Design review of the part built by this model. Coordinates are the model's own, in mm. Face numbers are marked on the shaded views. A direction names the side the tool comes from. Give positions to 0.01 mm unless a question says otherwise; leave off trailing zeros. Order: outer loops, then holes, each group sorted by start corner. A loop starts at its lowest first (then second) coordinate and runs counter-clockwise, first axis right, second up. Notation, with made-up numbers: (60, 34.25) -> (84, 34.25) arc R15 cw to (84, 54.25) -> close; hole circle Ø2 at (-39.75, 46.25). An arc over 180 degrees is marked (long way). Answer in a Markdown table with one row per item. Add a question column.
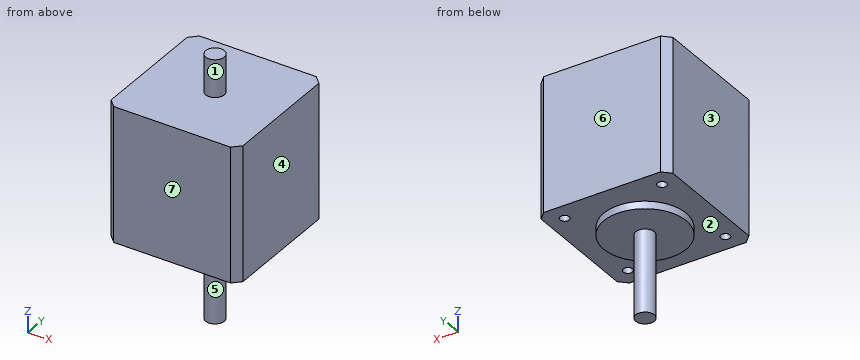
Solid Edge part; units mm, degrees
sketch "Sketch1" plane through (0, 0, 0) normal (0, 0, 1) x (1, 0, 0)
  circle A0 centre (0, 0) radius 2.5
extrude "Protrusion1" add sketch "Sketch1" along normal blind 24
sketch "Sketch2" plane through (0, 0, 24) normal (0, 0, 1) x (1, 0, 0)
  circle A0 centre (0, 0) radius 11
extrude "ExtrudedProtrusion_2" add sketch "Sketch2" against normal blind 2
sketch "Sketch3" plane through (0, 0, 24) normal (0, 0, 1) x (1, 0, 0)
  line L0 (-15.6, -17.6) -> (15.6, -17.6)
  line L1 (15.6, -17.6) -> (17.6, -15.6)
  line L2 (17.6, -15.6) -> (17.6, 15.6)
  line L3 (15.6, 17.6) -> (17.6, 15.6)
  line L4 (15.6, 17.6) -> (-15.6, 17.6)
  line L5 (-15.6, 17.6) -> (-17.6, 15.6)
  line L6 (-17.6, 15.6) -> (-17.6, -15.6)
  line L7 (-15.6, -17.6) -> (-17.6, -15.6)
extrude "ExtrudedProtrusion_3" add sketch "Sketch3" along normal blind 36
hole "Hole_1" at (-13, -13, 24) direction (0, 0, 1) diameter 2.459 depth 2.5 thread major 3 thread length 2.5
hole "Hole1" at (-13, 13, 24) direction (0, 0, 1) diameter 2.459 depth 2.5 thread major 3 thread length 2.5
hole "Hole2" at (13, 13, 24) direction (0, 0, 1) diameter 2.459 depth 2.5 thread major 3 thread length 2.5
hole "Hole3" at (13, -13, 24) direction (0, 0, 1) diameter 2.459 depth 2.5 thread major 3 thread length 2.5
sketch "Sketch4" plane through (0, 0, 60) normal (0, 0, 1) x (1, 0, 0)
  circle A0 centre (0, 0) radius 2.5
extrude "ExtrudedProtrusion_4" add sketch "Sketch4" along normal blind 10
1) Add section A-A, the plane x = -13. Write out the cut boundary in (y, z).
2) Clearance check with flat-ended pins moving along their axes: P1, Ø3, axis at x = 13, y = 13, coming from the -Z side; P2, Ø6.5, axis at x = 2, y = -3, coming from the -Z side; P3, Ø2, axis at x = -13, y = 13, coming from the +Z side; P4, Ø1.2, axis at x = 13, y = -13.5, coming from the -Z side. State where each tip first meets the part, or that it passes through.
3) Machinability: for the marked faces 1, 2 and 3, which of the approach directions +Z, -Z, +X, -X, +Y, -Y give a long, thin tool a straight path to every point of the face, cutting with its end or side? Answer none if there is none.
4) For L1, parallel to X at y = -13, z = 25.25; L2, parallel to Z at x = -13.5, y = 14.5, list the stretches that pass through material, from the lowest coordinate up.
5) Mouldability with a two-part tool opening along Y and no side actions: class the marked faces 4, 5, 6 and 7 as +Y half, -Y half, draft (parallel to the pull), parting line (faces both ways), or undercut.
6) Add section C-C, the plane z = 17. Write out the cut boundary in (x, y), and give its area (3 significant figures).
7) Add section D-D, the plane y = 0. Write out the cut boundary in (x, z).
Verdict:
| question | item | result |
|---|---|---|
| 1 | outline | (-17.6, 24) -> (-14.23, 24) -> (-14.23, 26.5) -> (-11.77, 26.5) -> (-11.77, 24) -> (11.77, 24) -> (11.77, 26.5) -> (14.23, 26.5) -> (14.23, 24) -> (17.6, 24) -> (17.6, 60) -> (-17.6, 60) -> close |
| 2 | P1 | stops at z = 24 |
| 2 | P2 | stops at z = 0 |
| 2 | P3 | stops at z = 60 |
| 2 | P4 | stops at z = 26.5 |
| 3 | face 1 | +Z |
| 3 | face 2 | -Z |
| 3 | face 3 | +Z, -Z, -X, +Y, -Y |
| 4 | L1 | x = -17.6 to -14.23, -11.77 to 11.77, 14.23 to 17.6 |
| 4 | L2 | z = 24 to 60 |
| 5 | face 4 | draft |
| 5 | face 5 | parting line |
| 5 | face 6 | +Y half |
| 5 | face 7 | -Y half |
| 6 | outline | circle Ø5 at (0, 0) |
| 6 | area | 19.6 mm2 |
| 7 | outline | (-17.6, 24) -> (-11, 24) -> (-11, 22) -> (-2.5, 22) -> (-2.5, 0) -> (2.5, 0) -> (2.5, 22) -> (11, 22) -> (11, 24) -> (17.6, 24) -> (17.6, 60) -> (2.5, 60) -> (2.5, 70) -> (-2.5, 70) -> (-2.5, 60) -> (-17.6, 60) -> close |
